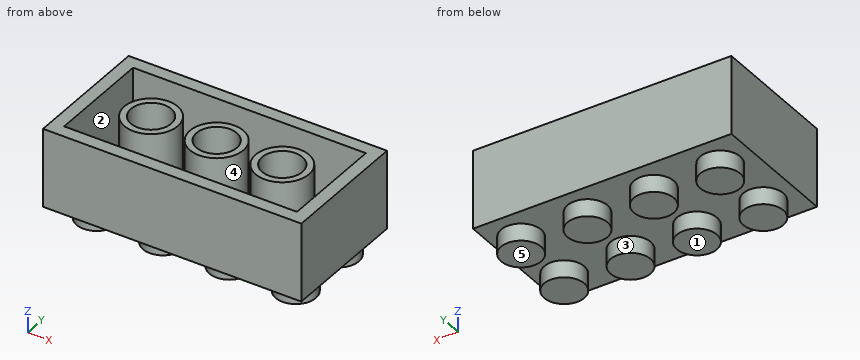
```python
from build123d import *

# Parameters (mm, degrees)
F0_W     = 31.548
F0_H     = 15.928
F0_W_2   = 28.434
F0_H_2   = 12.814
F1_DEPTH = 9.6
F2_DEPTH = 25
F3_DEPTH = 1.557
F4_R     = 3.267
F4_R_2   = 2.467
F5_DEPTH = 8.043
F6_R     = 2.45
F7_DEPTH = 2.1


with BuildPart() as f1:
    # F0 (on Top) → F1 (new body)
    with BuildSketch(Plane.XY):
        with Locations((-21.131882, -12.566023)):
            Rectangle(F0_W, F0_H)
        with Locations((-21.131882, -12.566023)):
            Rectangle(F0_W_2, F0_H_2, mode=Mode.SUBTRACT)
        with Locations((-21.131882, -12.566023)):
            Rectangle(F0_W_2, F0_H_2)
    extrude(amount=F1_DEPTH)

    # F0 (on Top) → F2 (cut)
    with BuildSketch(Plane.XY):
        with Locations((-21.131882, -12.566023)):
            Rectangle(F0_W_2, F0_H_2)
    extrude(amount=F2_DEPTH, mode=Mode.SUBTRACT)

    # F0 (on Top) → F3 (join)
    with BuildSketch(Plane.XY):
        with Locations((-21.131882, -12.566023)):
            Rectangle(F0_W_2, F0_H_2)
    extrude(amount=F3_DEPTH)

    # F4 (on face) → F5 (join)
    with BuildSketch(Plane.XY.offset(1.557)):
        with Locations((-28.941882, -12.566023)):
            Circle(F4_R)
        with Locations((-28.941882, -12.566023)):
            Circle(F4_R_2, mode=Mode.SUBTRACT)
        with Locations((-20.927882, -12.566023)):
            Circle(F4_R)
        with Locations((-20.927882, -12.566023)):
            Circle(F4_R_2, mode=Mode.SUBTRACT)
        with Locations((-12.913882, -12.566023)):
            Circle(F4_R)
        with Locations((-12.913882, -12.566023)):
            Circle(F4_R_2, mode=Mode.SUBTRACT)
    extrude(amount=F5_DEPTH)

    # F6 (on face) → F7 (join)
    with BuildSketch(Plane(origin=(0, 0, 0), x_dir=(1, 0, 0), z_dir=(0, 0, -1))):
        with Locations((-32.948882, 16.573023)):
            Circle(F6_R)
        with Locations((-24.844882, 16.573023)):
            Circle(F6_R)
        with Locations((-16.740882, 16.573023)):
            Circle(F6_R)
        with Locations((-8.636882, 16.573023)):
            Circle(F6_R)
        with Locations((-8.636882, 8.559023)):
            Circle(F6_R)
        with Locations((-16.740882, 8.559023)):
            Circle(F6_R)
        with Locations((-24.844882, 8.559023)):
            Circle(F6_R)
        with Locations((-32.948882, 8.559023)):
            Circle(F6_R)
    extrude(amount=F7_DEPTH)


solid = f1.part
```
The model under review builds one solid part; all positions refer to its coordinate system, in mm. Face numbers are marked on the shaded views. A direction names the side the tool comes from. Round coordinates to 2 decimals unless told otherwise and drop trailing zeros. Order: outer loops, then holes, each group sorted by start corner. A loop starts at its lowest first (then second) coordinate and runs counter-clockwise, first axis right, second up. Notation, with made-up numbers: (27.5, 72) -> (66.5, 72) arc R32 ccw to (66.5, 99) -> close; hole circle Ø4 at (1.5, 20.5). An arc over 180 degrees is marked (long way). One line per item, written item: value. Start each with the question number.
Q1. Take a section at D-D (x = -22). Write out the cut boundary in (y, z).
Q2. Machinability: for the marked faces 1, 2 and 3, which of the approach directions +Z, -Z, +X, -X, +Y, -Y give a long, thin tool a straight path to every point of the face, cutting with its end or side? Answer none if there is none.
Q3. Take a section at B-B (x = -29.5). Write out the cut boundary in (y, z) (3 decimals).
Q4. Mouldability with a two-part tool opening along Y and no side actions: class the marked faces 4 and 5 as released by +Y, released by -Y, zero draft, split by the parting line, or undercut.
Q5. Clearance check with a flat-ended pin moving along its axis: pin 1 Ø1.5 at (x, y) = (-28.5, -12.5) entering from +Z. State where the tip first meets the part, or that it passes through.
Q6. Wall thickness on line 1 (X direction, y = -8, z = 1.75); line 2 (X direction, y = -15.25, z = 1.75); line 3 (Y direction, x = -31, z = 6.25): over which ranges is each line inside the solid? List them lowest first.
Q7. Take a section at A-A (z = 6.75). Write out the cut boundary in (x, y).
Reported:
1. outline: (-20.53, 0) -> (-4.6, 0) -> (-4.6, 9.6) -> (-6.16, 9.6) -> (-6.16, 1.56) -> (-9.48, 1.56) -> (-9.48, 9.6) -> (-10.34, 9.6) -> (-10.34, 1.56) -> (-14.79, 1.56) -> (-14.79, 9.6) -> (-15.65, 9.6) -> (-15.65, 1.56) -> (-18.97, 1.56) -> (-18.97, 9.6) -> (-20.53, 9.6) -> close
2. face 1: -Z, +X, -X, +Y, -Y
2. face 2: +Z
2. face 3: -Z
3. outline: (-20.53, 0) -> (-4.602, 0) -> (-4.602, 9.6) -> (-6.159, 9.6) -> (-6.159, 1.557) -> (-9.347, 1.557) -> (-9.347, 9.6) -> (-10.163, 9.6) -> (-10.163, 1.557) -> (-14.969, 1.557) -> (-14.969, 9.6) -> (-15.785, 9.6) -> (-15.785, 1.557) -> (-18.973, 1.557) -> (-18.973, 9.6) -> (-20.53, 9.6) -> close
4. face 4: undercut
4. face 5: zero draft
5. pin 1: stops at z = 1.56
6. line 1: x = -36.91 to -35.35, -6.91 to -5.36
6. line 2: x = -36.91 to -35.35, -30.8 to -27.08, -22.79 to -19.07, -14.78 to -11.05, -6.91 to -5.36
6. line 3: y = -20.53 to -18.97, -15.1 to -13.93, -11.21 to -10.03, -6.16 to -4.6
7. outline: (-36.91, -20.53) -> (-5.36, -20.53) -> (-5.36, -4.6) -> (-36.91, -4.6) -> close; circle Ø6.53 at (-28.94, -12.57); circle Ø6.53 at (-20.93, -12.57); circle Ø6.53 at (-12.91, -12.57); hole (-35.35, -18.97) -> (-6.91, -18.97) -> (-6.91, -6.16) -> (-35.35, -6.16) -> close; hole circle Ø4.93 at (-28.94, -12.57); hole circle Ø4.93 at (-20.93, -12.57); hole circle Ø4.93 at (-12.91, -12.57)
